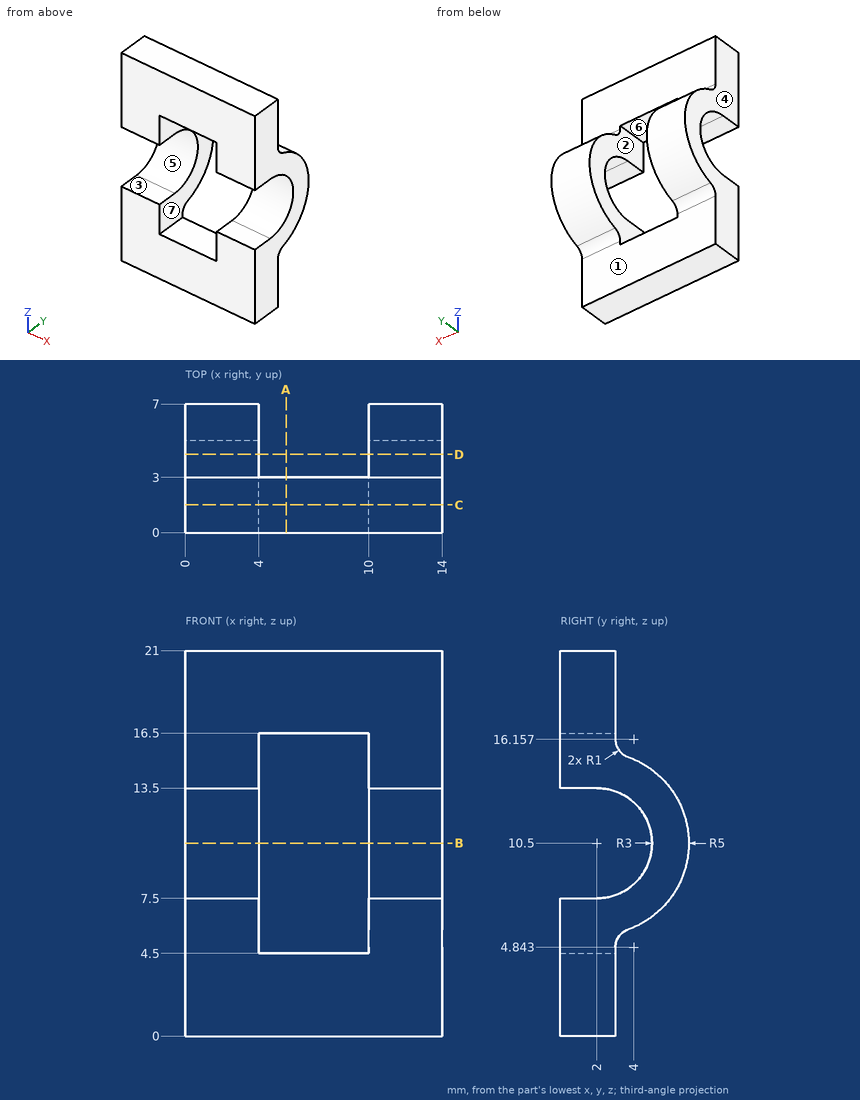
Input: dimensioned drawing with shaded views. Units: mm. Origin: part minimum x, y, z. A direction names the side the tool comes from. Give positions to 0.01 mm unless a question says otherwise; leave off trailing zeros. Write each loop counter-clockwise with the first axis right and the second up, starting at its lowest first coordinate (ties: lowest second). Pieces come first, ordered by that corner, then holes. Notation, with made-up numbers: (69, 14.25) - (117, 14.25) arc R21 ccw to (117, 29.25) - close; hole circle Ø10 at (33.25, 59.25). An arc over 180 degrees is marked (long way). Write item = value, one per line. Start each with the question number.
1) Material intervals for L1, parallel to Z at x = 3.5, y = 1; L2, parallel to Z at x = 4.25, y = 1; L3, parallel to X at y = 0.5, z = 6.25, sorted ascending. Write a range as [from, to].
2) Cut plane D-D (y = 4.25). Return loops of the section in (x, z) (1 decimal), and give its area (3 significant figures).
3) Pin query (flat end, axial travel): pin 1 (1.5 mm diameter, centred on x = 12.5, z = 11, fed in from -Y); pin 2 (1.6 mm diameter, centred on x = 1, y = 1, fed in from -Z); pin 3 (1.5 mm diameter, centred on x = 1.5, y = 4, fed in from -Z) (1 decimal); pin 4 (5.5 mm diameter, centred on x = 3.5, z = 2, fed in from +Y). Return the tip coordinate at first contact, or that it passes through.
4) Cut plane C-C (y = 1.5). Return loops of the section in (x, z), and give its area (3 significant figures).
5) Cut plane B-B (z = 10.5). Return loops of the section in (x, y).
6) Draft query along X for the marked faces 4, 5, 6 and 7. Return one class per face: pulls with the +X half, pulls with the -X half, needs draft (parallel to the pull), parting line crosses it, or undercut.
7) Cut plane A-A (x = 5.5). Return loops of the section in (y, z), and give its area (3 significant figures).
8) Reachability of the marked faces 1, 2 and 3 from +Z, -Z, +X, -X, +Y, -Y: full face, straight path, thin tool, end or side. Return the list, or none.
Answers follow:
q1.L1 = [0, 7.5], [13.5, 21]
q1.L2 = [0, 4.5], [16.5, 21]
q1.L3 = [0, 4], [10, 14]
q2.outline = (0, 6) - (4, 6) - (4, 8.5) - (0, 8.5) - close; (0, 12.5) - (4, 12.5) - (4, 15) - (0, 15) - close; (10, 6) - (14, 6) - (14, 8.5) - (10, 8.5) - close; (10, 12.5) - (14, 12.5) - (14, 15) - (10, 15) - close
q2.area = 39.7 mm^2
q3.pin_1 = 4.73
q3.pin_2 = 0
q3.pin_3 = 5.5
q3.pin_4 = 3
q4.outline = (0, 0) - (14, 0) - (14, 7.5) - (10, 7.5) - (10, 4.5) - (4, 4.5) - (4, 7.5) - (0, 7.5) - close; (0, 13.5) - (4, 13.5) - (4, 16.5) - (10, 16.5) - (10, 13.5) - (14, 13.5) - (14, 21) - (0, 21) - close
q4.area = 174 mm^2
q5.outline = (0, 5) - (4, 5) - (4, 7) - (0, 7) - close; (10, 5) - (14, 5) - (14, 7) - (10, 7) - close
q6.face_4 = pulls with the -X half
q6.face_5 = needs draft
q6.face_6 = undercut
q6.face_7 = undercut
q7.outline = (0, 0) - (3, 0) - (3, 4.5) - (0, 4.5) - close; (0, 16.5) - (3, 16.5) - (3, 21) - (0, 21) - close
q7.area = 27.0 mm^2
q8.face_1 = -Z, +X, -X, +Y
q8.face_2 = +Y, -Y
q8.face_3 = +X, -X, -Y
